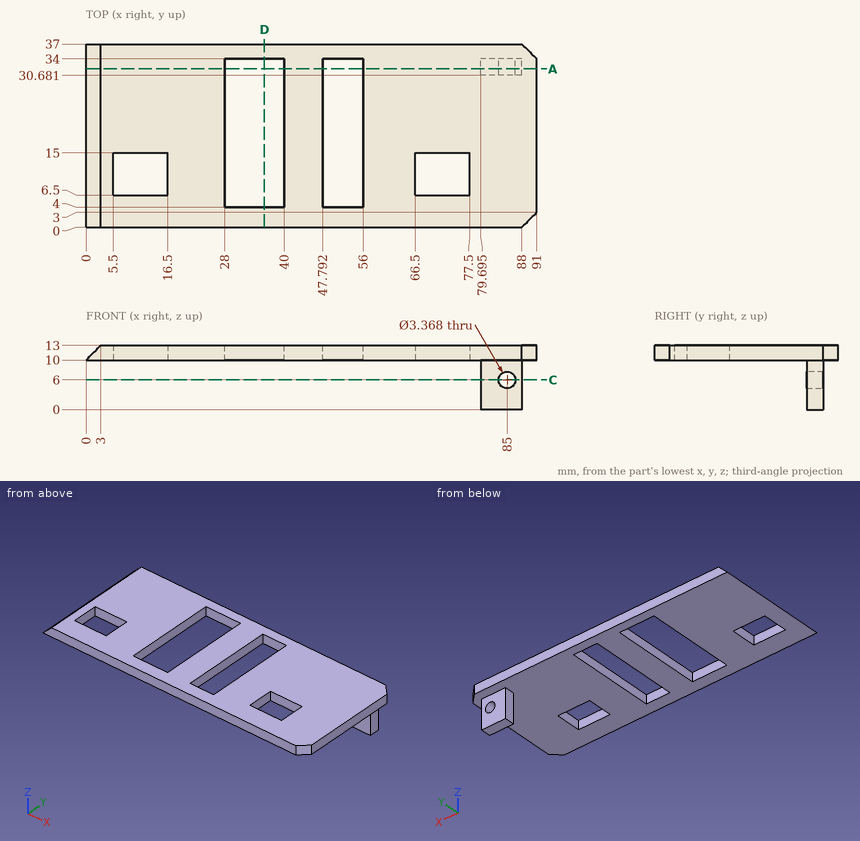
Part print with two shaded views. Sizes in mm from the minimum x, y, z corner. Give positions to 0.01 mm unless a question says otherwise; leave off trailing zeros. Order: outer loops, then holes, each group sorted by start corner. A loop starts at its lowest first (then second) coordinate and runs counter-clockwise, first axis right, second up. Notation, with made-up numbers: M -11,64.5 L 40,64.5 A22 ccw 40,70.5 Z; hole C 63,42 d5. An arc over 180 degrees is marked long. Write item = value, one per line.
Q1. Cut at C-C, the plane z = 6. List the corners of the cut face in (x, y) (1 decimal), then the cut area to 3 significant figures.
Derived:
outline = M 79.7,30.7 L 83.3,30.7 L 83.3,34 L 79.7,34 Z; M 86.7,30.7 L 88,30.7 L 88,34 L 86.7,34 Z
area = 16.4 mm2
Q2. Cut at D-D, the plane x = 36. List the corners of the cut face in (y, z), then the cut area to 3 significant figures.
Derived:
outline = M 0,10 L 4,10 L 4,13 L 0,13 Z; M 34,10 L 37,10 L 37,13 L 34,13 Z
area = 21.0 mm2
Q3. Flat gauge pins, fed straight in: pin 1 (1.7 mm diameter, centred on y = 32.5, z = 3.5, fed in from -X) (1 decimal); pin 2 (12 mm diameter, centred on x = 15, y = 18, fed in from -Z); pin 3 (4 mm diameter, centred on x = 83, z = 4.5, fed in from -Y); pin 4 (10 mm diameter, centred on x = 38, y = 8, fed in from +Z). Where does each tip first touch, or does it go through?
Derived:
pin_1 = 79.7
pin_2 = 10
pin_3 = 30.68
pin_4 = 13
Q4. Cut at A-A, the plane y = 32. Count the separate pieces of the cut face and the enclosed holes in it, then the cut area to 3 significant figures.
Derived:
separate_pieces = 3
enclosed_holes = 1
area = 282 mm2
Q5. Drill centre lines: line 1 (Y direction, x = 53.5, z = 11.25); line 2 (Z direction, x = 85, y = 31.6); line 3 (X direction, y = 32.65, z = 6) (1 decimal). Where is each one in solid material? Low to high. Write a range as [from, to].
Derived:
line_1 = [0, 4], [34, 37]
line_2 = [0, 4.32], [7.68, 13]
line_3 = [79.7, 83.3], [86.7, 88]
